Source: CAD feature listing. Evaluate the final solid. Frame: model axes, mm. A direction names the side the tool comes from. Round coordinates to 2 decimals unless told otherwise and drop trailing zeros. Order: outer loops, then holes, each group sorted by start corner. A loop starts at its lowest first (then second) coordinate and runs counter-clockwise, first axis right, second up. Notation, with made-up numbers: (-9, -20) - (8, -20) arc R25 ccw to (8, 19) - close; hole circle Ø2 at (-30.5, 48.5). An arc over 180 degrees is marked (long way). Return JSON: item names as keys, results as strings. Group by question number.
1) Section C-C, the plane y = 21. Return loops of the section in (x, z), plus the area to 3 significant figures.
2) Section A-A, the plane y = 0. Return loops of the section in (x, z).
3) Mould query, pull axis Y, two halves, no side actions, for faces 1 (the flat face through (1, 30, 29)), 2 (the cylindrical face through (1.265, -27.042, 56.403)), 3 (the flat face through (-1, -24, 40)), 4 (the flat face through (27.5, 0, 32)). Classes: pulls with the +Y half, pulls with the -Y half, needs draft (parallel to the pull), parting line crosses it, or undercut.
4) Section B-B, the plane z = 37.5. Return loops of the section in (x, y).
5) Contact query for flat-ended pins moving along their axis: P1, Ø4, axis at y = 12, z = 2, coming from the -X side; P2, Ø10, axis at x = -5, z = 6.5, coming from the +Y side; P3, Ø1.5, axis at x = 54.5, y = -4, coming from the +Z side; P4, Ø8, axis at x = -81, y = 11.5, coming from the -Z side. Output: stop coordinate, or through.
6) Section D-D, the plane x = -7.5. Return loops of the section in (y, z), plus the area to 3 significant figures.
7) Access query for faces 5 (the cylindrical face through (-34, 0, 13)), 6 (the flat face through (80, 0, 10)), 7 (the flat face through (0, -10, 25)), 8 (the flat face through (-27.5, 0, 32)). Directions: +Z, -Z, +X, -X, +Y, -Y. A direction counts if a zero-diameter tool reaches every point of the face in a straight line with its end or side. Return the directions, or none.
8) Ray query, line 1 (Y direction, x = 3.5, z = 20); line 2 (Y direction, x = 10, z = 41); line 3 (X direction, y = -0.5, z = 26.5). Return the intervals inside material, ascending. Write a range as from..to.
```python
from build123d import *

# Parameters (mm, degrees)
F0_W      = 170
F0_H      = 60
F1_DEPTH  = 30
F3_DEPTH  = 30.001
F5_DEPTH  = 60.001
F6_W      = 55
F6_H      = 48
F7_DEPTH  = 5
F8_DEPTH  = 25
F10_DEPTH = 60.001
F13_DEPTH = 6
F14_DEPTH = 6
F17_DEPTH = 6


with BuildPart() as f1:
    # F0 (on Top) → F1 (new body)
    with BuildSketch(Plane.XY):
        Rectangle(F0_W, F0_H)
    extrude(amount=F1_DEPTH)

    # F2 (on face) → F3 (cut, through all)
    with BuildSketch(Plane.XY.offset(30)):
        with BuildLine():
            ThreePointArc((0, 0), (2.9289321881, -7.0710678119), (10, -10))
            Line((10, -10), (10, 10))
            ThreePointArc((10, 10), (2.9289321881, 7.0710678119), (0, 0))
        make_face()
        with BuildLine():
            Line((-10, -10), (10, -10))
            ThreePointArc((10, -10), (2.9289321881, -7.0710678119), (0, 0))
            ThreePointArc((0, 0), (-2.9289321881, -7.0710678119), (-10, -10))
        make_face()
        with BuildLine():
            Line((10, 10), (10, -10))
            ThreePointArc((10, -10), (17.0710678119, -7.0710678119), (20, 0))
            ThreePointArc((20, 0), (17.0710678119, 7.0710678119), (10, 10))
        make_face()
        with BuildLine():
            ThreePointArc((-10, 10), (-20, 0), (-10, -10))
            Line((-10, -10), (-10, 10))
        make_face()
        with BuildLine():
            Line((-10, 10), (-10, -10))
            ThreePointArc((-10, -10), (-2.9289321881, -7.0710678119), (0, 0))
            ThreePointArc((0, 0), (-2.9289321881, 7.0710678119), (-10, 10))
        make_face()
        with BuildLine():
            ThreePointArc((0, 0), (2.9289321881, 7.0710678119), (10, 10))
            Line((10, 10), (-10, 10))
            ThreePointArc((-10, 10), (-2.9289321881, 7.0710678119), (0, 0))
        make_face()
    extrude(amount=-F3_DEPTH, mode=Mode.SUBTRACT)

    # F4 (on face) → F5 (cut, through all)
    with BuildSketch(Plane(origin=(0, 30, 0), x_dir=(-1, 0, 0), z_dir=(0, 1, 0))):
        with BuildLine():
            Line((-35, 0), (0, 0))
            Line((0, 0), (35, 0))
            Line((35, 0), (35, 10))
            ThreePointArc((35, 10), (33.5355339059, 13.5355339059), (30, 15))
            Line((30, 15), (-30, 15))
            ThreePointArc((-30, 15), (-33.5355339059, 13.5355339059), (-35, 10))
            Line((-35, 10), (-35, 0))
        make_face()
    extrude(amount=-F5_DEPTH, mode=Mode.SUBTRACT)

    # F6 (on face) → F7 (join)
    with BuildSketch(Plane.XY.offset(30)):
        Rectangle(F6_W, F6_H)
    extrude(amount=F7_DEPTH)

    # F8 (cut): a face of the model
    f8_faces = [f1.faces().sort_by_distance(p)[0] for p in [
        (0, 0, 30),
    ]]
    extrude(f8_faces, amount=-F8_DEPTH, mode=Mode.SUBTRACT)

    # F9 (on face) → F10 (cut, through all)
    with BuildSketch(Plane(origin=(0, 30, 0), x_dir=(-1, 0, 0), z_dir=(0, 1, 0))):
        with BuildLine():
            Line((85, 0), (85, 10))
            Line((85, 10), (75, 10))
            ThreePointArc((75, 10), (71.4644660941, 8.5355339059), (70, 5))
            Line((70, 5), (70, 0))
            Line((70, 0), (85, 0))
        make_face()
        with BuildLine():
            Line((-85, 10), (-85, 0))
            Line((-85, 0), (-70, 0))
            Line((-70, 0), (-70, 5))
            ThreePointArc((-70, 5), (-71.4644660941, 8.5355339059), (-75, 10))
            Line((-75, 10), (-85, 10))
        make_face()
    extrude(amount=-F10_DEPTH, mode=Mode.SUBTRACT)

    # F12 (on face) → F13 (join)
    with BuildSketch(Plane.XZ.offset(30)):
        with BuildLine():
            Line((-85, 30), (85, 30))
            ThreePointArc((85, 30), (0, 56.4079290569), (-85, 30))
        make_face()
    extrude(amount=-F13_DEPTH)

    # F16 (on face) → F17 (join)
    with BuildSketch(Plane(origin=(0, 30, 0), x_dir=(-1, 0, 0), z_dir=(0, 1, 0))):
        with BuildLine():
            Line((-85, 30), (85, 30))
            ThreePointArc((85, 30), (0, 56.4079290569), (-85, 30))
        make_face()
    extrude(amount=-F17_DEPTH)


with BuildPart() as f14:
    # F11 (on face) → F14 (new body)
    with BuildSketch(Plane(origin=(0, 30, 0), x_dir=(-1, 0, 0), z_dir=(0, 1, 0))):
        with BuildLine():
            Line((-85, 30), (85, 30))
            ThreePointArc((85, 30), (0, 56.4079290569), (-85, 30))
        make_face()
    extrude(amount=-F14_DEPTH)


solid = f1.part
```
Geometry check:
{
 "1": {"outline": "(-85, 10) - (-75, 10) arc R5 cw to (-70, 5) - (-70, 0) - (-35, 0) - (-35, 10) arc R5 cw to (-30, 15) - (30, 15) arc R5 cw to (35, 10) - (35, 0) - (70, 0) - (70, 5) arc R5 cw to (75, 10) - (85, 10) - (85, 30) - (27.5, 30) - (27.5, 35) - (-27.5, 35) - (-27.5, 30) - (-85, 30) - close", "area": "4,050 mm2"},
 "2": {"outline": "(-85, 10) - (-75, 10) arc R5 cw to (-70, 5) - (-70, 0) - (-35, 0) - (-35, 10) arc R5 cw to (-30, 15) - (-20, 15) - (-20, 35) - (-27.5, 35) - (-27.5, 30) - (-85, 30) - close; (20, 15) - (30, 15) arc R5 cw to (35, 10) - (35, 0) - (70, 0) - (70, 5) arc R5 cw to (75, 10) - (85, 10) - (85, 30) - (27.5, 30) - (27.5, 35) - (20, 35) - close"},
 "3": {"face 1": "pulls with the +Y half", "face 2": "needs draft", "face 3": "undercut", "face 4": "undercut"},
 "4": {"outline": "(-72.9, -30) - (72.9, -30) - (72.9, -24) - (-72.9, -24) - close; (-72.9, 24) - (72.9, 24) - (72.9, 30) - (-72.9, 30) - close"},
 "5": {"P1": "x = -70", "P2": "through", "P3": "z = 30", "P4": "z = 10"},
 "6": {"outline": "(-30, 15) - (-10, 15) - (-10, 35) - (-24, 35) - (-24, 56.22) - (-30, 56.22) - close; (10, 15) - (30, 15) - (30, 56.22) - (24, 56.22) - (24, 35) - (10, 35) - close", "area": "1,050 mm2"},
 "7": {"face 5": "-Z, +Y, -Y", "face 6": "-Z, +X, +Y, -Y", "face 7": "+Z, -Z", "face 8": "+Z, -X"},
 "8": {"line 1": "-30..-10, 10..30", "line 2": "-30..-24, 24..30", "line 3": "-85..-19.99, 19.99..85"}
}
